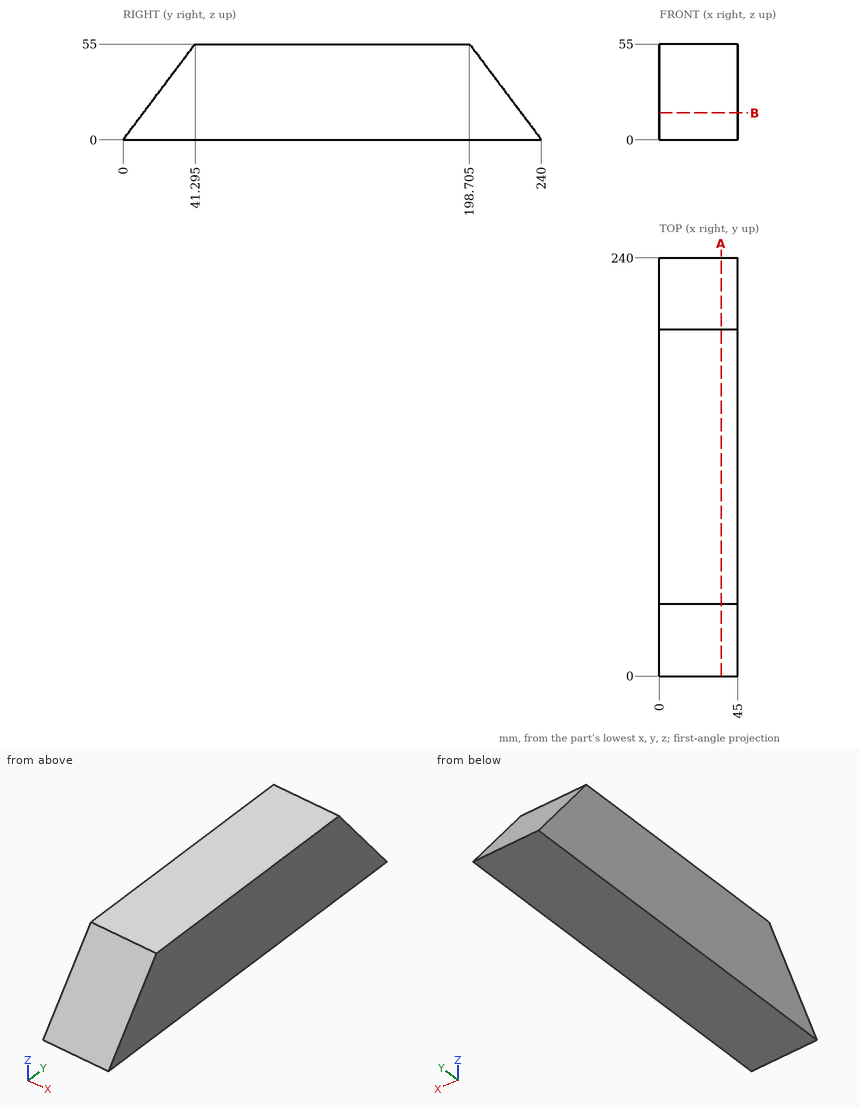
The figure shows three views and two pictorial views of one solid part (mm, origin at its lowest corner). Answer the questions. Coordinates: 2 decimals unless noted, no trailing zeros. Loops run counter-clockwise (first coordinate to the right, second up) from the corner with the lowest first, then second, coordinate; pieces in that order, holes last. Notation, with made-up numbers: (78, -10) - (95, -10) arc R36 cw to (95, 27) - close; hole circle Ø11 at (-30, -33). An arc over 180 degrees is marked (long way). Use a Markdown table: item, result. Add a question column.
1) Find the intervals of material crossed by line 1 (Z direction, x = 25, y = 209); line 2 (Z direction, x = 31, y = 221.5); line 3 (Y direction, x = 17.5, z = 22.5), in increasing order.
2) The part is cut by section B-B, the plane z = 15.5. Give the vertices of the cut face in (x, y).
3) The part is cut by section A-A, the plane x = 35.5. Give the vertices of the cut face in (y, z) (1 decimal), and give its area (3 significant figures).
4) Given pin 1 (3 mm diameter, centred on x = 14, y = 171.5, fed in from -Z); pin 2 (12 mm diameter, centred on x = 27, z = 21, fed in from +Y); pin 3 (8 mm diameter, centred on x = 34, y = 27.5, fed in from +Z); pin 4 (1 mm diameter, centred on x = 8, z = 43, fed in from -Y), each flat-ended and moving along its own axis, determine where each tip first touches the part or whether it passes through.
Here are the results:
| question | item | result |
|---|---|---|
| 1 | line 1 | z = 0 to 41.29 |
| 1 | line 2 | z = 0 to 24.64 |
| 1 | line 3 | y = 16.89 to 223.11 |
| 2 | outline | (0, 11.64) - (45, 11.64) - (45, 228.36) - (0, 228.36) - close |
| 3 | outline | (0, 0) - (240, 0) - (198.7, 55) - (41.3, 55) - close |
| 3 | area | 10,900 mm^2 |
| 4 | pin 1 | stops at z = 0 |
| 4 | pin 2 | stops at y = 228.74 |
| 4 | pin 3 | stops at z = 41.95 |
| 4 | pin 4 | stops at y = 31.91 |
